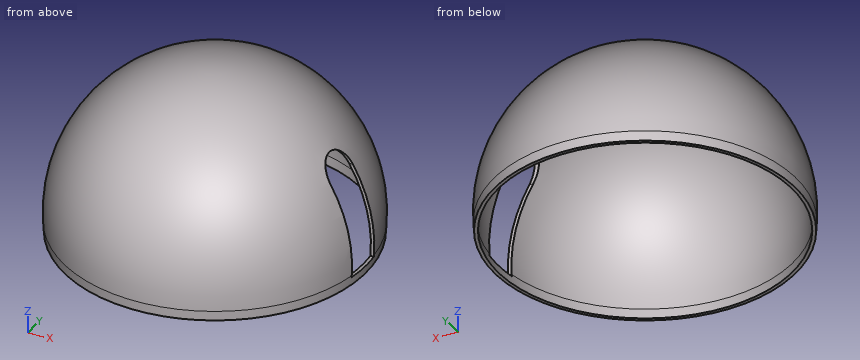
```python
from build123d import *

# Parameters (mm, degrees)
CUT_EXTRUDE1_DEPTH = 37.631109163


with BuildPart() as part:
    # Sketch2 → Revolve1 (revolve)
    with BuildSketch(Plane(origin=(0, -7.374853929, -7.41), x_dir=(-1, 0, 0), z_dir=(0, -1, 0))):
        with BuildLine():
            Line((50.149352541, -7.41), (50.339283308, -10.312639962))
            ThreePointArc((50.339283308, -10.312639962), (38.805254547, -42.539770141), (7.4, -56.153429675))
            Line((7.4, -56.153429675), (7.4, -57.153429675))
            ThreePointArc((7.4, -57.153429675), (39.535081297, -43.22340229), (51.337149367, -10.247345792))
            Line((51.337149367, -10.247345792), (51.151491045, -7.41))
            Line((51.151491045, -7.41), (50.149352541, -7.41))
        make_face()
    revolve(axis=Axis((-7.4, -7.374853929, -2), (0, 0, 1)))

    # Sketch3 → Cut-Extrude1 (cut, through all)
    with BuildSketch(Plane(origin=(0, 0, 0), x_dir=(0, 0, -1), z_dir=(1, 0, 0))):
        with BuildLine():
            Line((-2.348097087, -13.16), (-28.25, -13.16))
            ThreePointArc((-28.25, -13.16), (-34, -7.41), (-28.25, -1.66))
            Line((-28.25, -1.66), (-2.348097087, -1.66))
            Line((-2.348097087, -1.66), (-2.348097087, -13.16))
        make_face()
    extrude(amount=CUT_EXTRUDE1_DEPTH, mode=Mode.SUBTRACT)


solid = part.part
```
Model file for the job. Use its own axes, mm. Coordinates: 2 decimals unless noted, no trailing zeros. Loops run counter-clockwise (first coordinate to the right, second up) from the corner with the lowest first, then second, coordinate; pieces in that order, holes last. Notation, with made-up numbers: (21, 71.5) - (25, 71.5) arc R6 ccw to (25, 80.5) - close; hole circle Ø8 at (10, 72.5). An arc over 180 degrees is marked (long way). Answer as a JSON object with one key per item and string values. Group by question number.
(1) Cut at A-A (x = -7.4). Give the cut face in (y, z).
(2) Probe line 1 along Y through (x, z) = (-17, 12.5); line 2 along X through (y, z) = (-10.5, 36.5); line 3 along X through (y, z) = (9, 20.5). List the from-to ranges inside material, lowest first.
(3) Cut at C-C (z = 7). Give the cut face in (x, y), then the cut area to 3 significant figures.
(4) Cut at B-B (z = 16). Give the cut face in (x, y).
(5) Flat gauge pins, fed straight in: pin 1 (2 mm diameter, centred on x = 33, z = 12, fed in from -Y); pin 2 (1 mm diameter, centred on x = 21, y = -8, fed in from +Z); pin 3 (3 mm diameter, centred on x = 25, z = 19, fed in from +Y). Where does each tip first touch, or does it go through?
Geometry says:
{
 "1": {"outline": "(-51.31, 2.84) - (-51.13, 0) - (-50.12, 0) - (-50.31, 2.9) arc R43.03 cw (long way) to (35.56, 2.9) - (35.37, 0) - (36.38, 0) - (36.56, 2.84) arc R44.03 ccw (long way) to start"},
 "2": {"line 1": "y = -49.81 to -48.77, 34.02 to 35.06", "line 2": "x = -38.72 to -37.3, 22.5 to 23.92", "line 3": "x = -45.5 to -44.34, 29.54 to 30.7"},
 "3": {"outline": "(35.22, -13.16) arc R43.01 cw (long way) to (35.23, -1.66) - (36.24, -1.66) arc R44.01 ccw (long way) to (36.23, -13.16) - close", "area": "262 mm^2"},
 "4": {"outline": "(33.98, -13.16) arc R41.78 cw (long way) to (33.99, -1.66) - (35.03, -1.66) arc R42.81 ccw (long way) to (35.02, -13.16) - close"},
 "5": {"pin 1": "stops at y = -26.02", "pin 2": "stops at z = 39.77", "pin 3": "stops at y = 21.18"}
}
